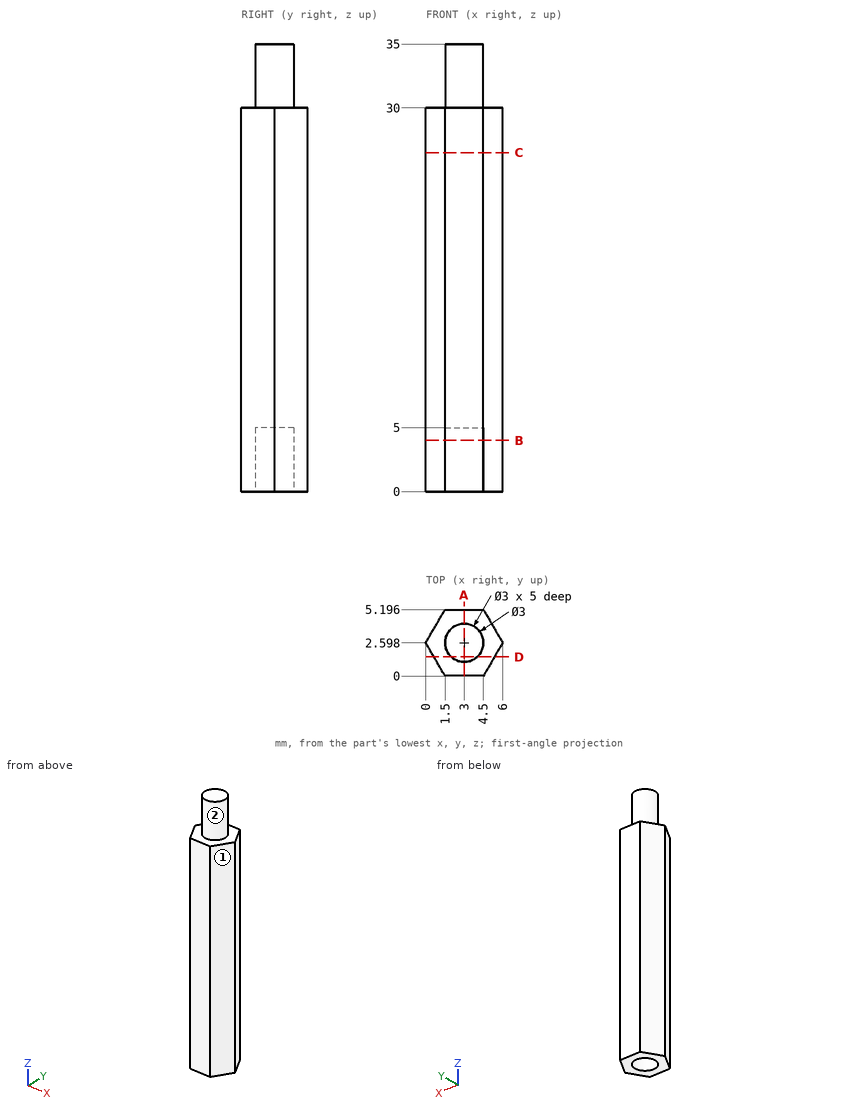
Geometry check sheet. Reference: drawing and pictorial views, mm from the part's lowest x, y, z. A direction names the side the tool comes from. Give positions to 0.01 mm unless a question says otherwise; leave off trailing zeros. Loops run counter-clockwise (first coordinate to the right, second up) from the corner with the lowest first, then second, coordinate; pieces in that order, holes last. Notation, with made-up numbers: (88.5, 18) - (126.5, 18) arc R6 cw to (126.5, 29) - close; hole circle Ø11 at (78, -4). An arc over 180 degrees is marked (long way). Use CSV: the item, a comma, the result in double quotes. Start each with the question number.
Q1. Access from +Z, -Z, +X, -X, +Y, -Y to the whole of each face (thin tool, end or side, straight path). Record for the marked faces 1 and 2.
Q2. Section check C-C, the plane z = 26.5. Record the cut outline in (x, y), and give its area (3 significant figures).
Q3. Section check D-D, the plane y = 1.5. Record the cut outline in (x, z), and give its area (3 significant figures).
Q4. Scan lines: probe 1 along Y at (x, z) = (3, 2.35); probe 2 along Z at (x, y) = (3.75, 0.45); probe 3 along Z at (x, y) = (3.8, 3.15). Record each from-to range of solid material in increasing order. Write a range as from..to.
Q5. Go/stop test with a flat-tipped pin: pin 1 Ø1.5 at (x, y) = (3.5, 3) entering from -Z. Record where the tip stops, or that it passes through.
Q6. Section check A-A, the plane x = 3. Record the cut outline in (y, z), and give its area (3 significant figures).
Q7. Section check B-B, the plane z = 4. Record the cut outline in (x, y), and give its area (3 significant figures).
Findings below:
1,face 1,"+Z, -Z, +X, -Y"
1,face 2,"+Z"
2,outline,"(0, 2.6) - (1.5, 0) - (4.5, 0) - (6, 2.6) - (4.5, 5.2) - (1.5, 5.2) - close"
2,area,"23.4 mm^2"
3,outline,"(0.63, 0) - (1.98, 0) - (1.98, 5) - (4.02, 5) - (4.02, 0) - (5.37, 0) - (5.37, 30) - (4.02, 30) - (4.02, 35) - (1.98, 35) - (1.98, 30) - (0.63, 30) - close"
3,area,"142 mm^2"
4,probe 1,"y = 0..1.1, 4.1..5.2"
4,probe 2,"z = 0..30"
4,probe 3,"z = 5..35"
5,pin 1,"stops at z = 5"
6,outline,"(0, 0) - (1.1, 0) - (1.1, 5) - (4.1, 5) - (4.1, 0) - (5.2, 0) - (5.2, 30) - (4.1, 30) - (4.1, 35) - (1.1, 35) - (1.1, 30) - (0, 30) - close"
6,area,"156 mm^2"
7,outline,"(0, 2.6) - (1.5, 0) - (4.5, 0) - (6, 2.6) - (4.5, 5.2) - (1.5, 5.2) - close; hole circle Ø3 at (3, 2.6)"
7,area,"16.3 mm^2"
